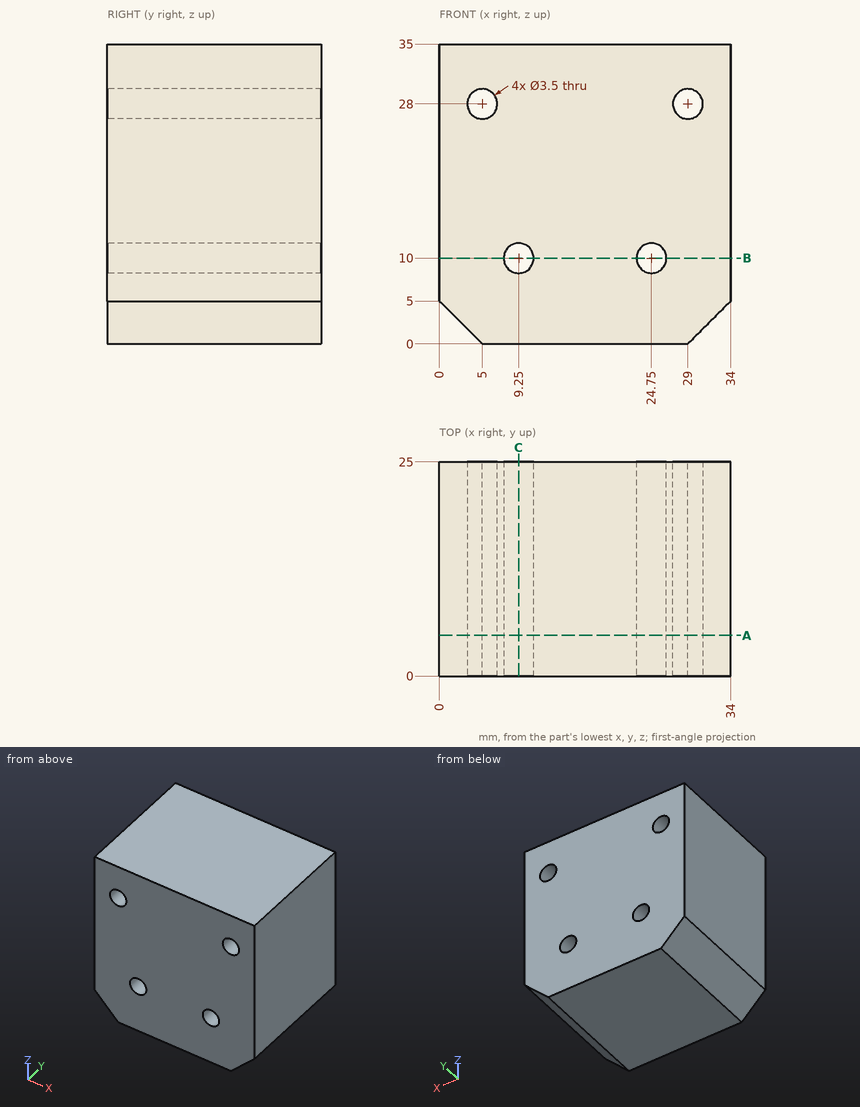
Design review of the part shown in the three views and the two pictorial views. Dimensions are in mm from the part's minimum x, y and z. Coordinates: 2 decimals unless noted, no trailing zeros. Loops run counter-clockwise (first coordinate to the right, second up) from the corner with the lowest first, then second, coordinate; pieces in that order, holes last.
(1) Consider section C-C, the plane x = 9.25. Give the boundary of the cut face in (y, z), plus the area to 4 significant figures.
Determined:
outline: (0, 0) - (25, 0) - (25, 8.25) - (0, 8.25) - close; (0, 11.75) - (25, 11.75) - (25, 35) - (0, 35) - close
area: 787.5 mm2
(2) Consider section B-B, the plane z = 10. Give the boundary of the cut face in (x, y), plus the area to 3 significant figures.
Determined:
outline: (0, 0) - (7.5, 0) - (7.5, 25) - (0, 25) - close; (11, 0) - (23, 0) - (23, 25) - (11, 25) - close; (26.5, 0) - (34, 0) - (34, 25) - (26.5, 25) - close
area: 675 mm2
(3) Insertion check: P1, Ø5.5, axis at x = 9.25, z = 10, coming from the +Y side; P2, Ø2, axis at x = 24.75, z = 10, coming from the +Y side. Each pin has a flat end and moves straight along its axis. Give the tip position at first contact, or say it passes through.
Determined:
P1: stops at y = 25
P2: passes through
(4) Consider section A-A, the plane y = 4.75. Give the boundary of the cut face in (x, z).
Determined:
outline: (0, 5) - (5, 0) - (29, 0) - (34, 5) - (34, 35) - (0, 35) - close; hole circle Ø3.5 at (5, 28); hole circle Ø3.5 at (9.25, 10); hole circle Ø3.5 at (24.75, 10); hole circle Ø3.5 at (29, 28)
(5) Wall thickness on L1, parallel to Z at x = 5, y = 15.25; L2, parallel to X at y = 6, z = 27.5; L3, parallel to Z at x = 28, y = 16.5: over which ranges is each line inside the solid? List them lowest first.
Determined:
L1: z = 0 to 26.25, 29.75 to 35
L2: x = 0 to 3.32, 6.68 to 27.32, 30.68 to 34
L3: z = 0 to 26.56, 29.44 to 35
